Work out the finished part from the listing and answer in its coordinate system (mm). Coordinates: 2 decimals unless noted, no trailing zeros. Order: outer loops, then holes, each group sorted by start corner. A loop starts at its lowest first (then second) coordinate and runs counter-clockwise, first axis right, second up. Notation, with made-up numbers: (-4, 70) -> (22, 70) arc R19 cw to (22, 106) -> close; hole circle Ø9 at (81, -30.5). An arc over 180 degrees is marked (long way). Answer as CSV lines item,"result". Start each with the question number.
Item 1: Section D-D (z = -280.5) is taken. Write down the section's boundary in (x, y), then the cut area to 3 significant figures.
Item 2: Each of these flat-tipped pins is pushed along its axis until it touches: pin 1 Ø2 at (x, z) = (333.5, 118.5) entering from -Y; pin 2 Ø0.5 at (x, y) = (-524.5, 37) entering from +Z; pin 3 Ø8 at (y, z) = (11.5, 20) entering from +X. Where does it stop, or does it pass through?
Item 3: Straight lines are drawn through the part: L1, parallel to Z at x = 0, y = 65; L2, parallel to Y at x = 367, z = 51; L3, parallel to X at y = 33.5, z = 119. For each, find the intervals that lie inside material, in ascending order.
Item 4: Section B-B (z = 28) is taken. Write down the section's boundary in (x, y).
Item 5: Section C-C (y = 22) is taken. Write down the section's boundary in (x, z) (1 decimal), then the cut area to 3 significant figures.
Item 6: Section A-A (x = 0) is taken. Write down the section's boundary in (y, z), then the cut area to 3 significant figures.
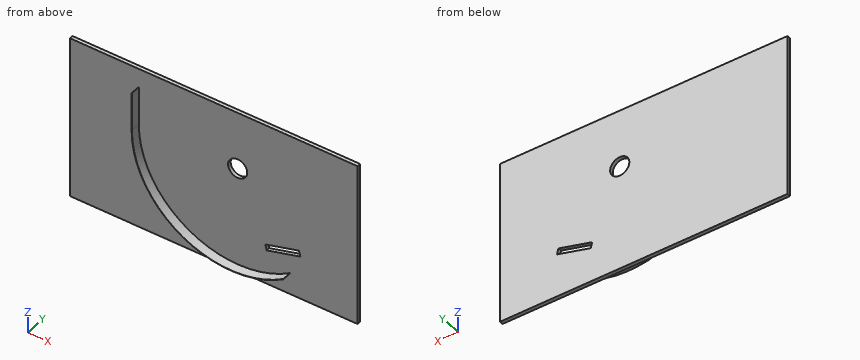
```python
from build123d import *

# Parameters (mm, degrees)
BOSS_EXTRUDE1_DEPTH    = 50.8
SKETCH4_W              = 1524
SKETCH4_H              = 863.6
BOSS_EXTRUDE2_DEPTH    = 19.05
F_20_0MM_DOWEL_HOLE1_D = 101.6
SKETCH8_W              = 1.5875
SKETCH8_H              = 50.8
BOSS_EXTRUDE3_DEPTH    = 204
CUT_EXTRUDE1_DEPTH     = 1052.265465998


with BuildPart() as part:
    # Sketch3 → Boss-Extrude1 (new body)
    with BuildSketch(Plane(origin=(0, 0, 0), x_dir=(1, 0, 0), z_dir=(0, 1, 0))):
        with BuildLine():
            Line((-524, 0), (-525.5875, 0))
            ThreePointArc((-525.5875, 0), (-255.243310314, 459.448661655), (277.677694458, 446.248045549))
            Line((277.677694458, 446.248045549), (277.677694458, 444.377202386))
            ThreePointArc((277.677694458, 444.377202386), (-254.040241009, 458.300726541), (-524, 0))
        make_face()
    extrude(amount=BOSS_EXTRUDE1_DEPTH)

    # Sketch4 → Boss-Extrude2 (add)
    with BuildSketch(Plane(origin=(0, 50.8, 0), x_dir=(1, 0, 0), z_dir=(0, 1, 0))):
        with Locations((-127, 127)):
            Rectangle(SKETCH4_W, SKETCH4_H)
    extrude(amount=BOSS_EXTRUDE2_DEPTH)

    # Ø20.0mm Dowel Hole1 (through all)
    with Locations(Plane(origin=(0, 50.8, 0), x_dir=(-1, 0, 0), z_dir=(0, -1, 0))):
        with Locations((0, 0)):
            Hole(F_20_0MM_DOWEL_HOLE1_D / 2)

    # Sketch8 → Boss-Extrude3 (add)
    with BuildSketch(Plane.XY):
        with Locations((-524.79375, 25.4)):
            Rectangle(SKETCH8_W, SKETCH8_H)
    extrude(amount=BOSS_EXTRUDE3_DEPTH)

    # Sketch9 → Cut-Extrude1 (cut, through all)
    with BuildSketch(Plane(origin=(0, 50.8, 0), x_dir=(-1, 0, 0), z_dir=(0, -1, 0))):
        Polygon((-154.06829349, 376.859298133), (-332.764571353, 328.977774789), (-325, 300), (-146.303722137, 347.881523344), align=None)
    extrude(amount=-CUT_EXTRUDE1_DEPTH, mode=Mode.SUBTRACT)


solid = part.part
```
Checked values:
1,outline,"(-889, 50.8) -> (-444.48, 50.8) -> (-444.48, 0) -> (-442.6, 0) -> (-442.6, 50.8) -> (635, 50.8) -> (635, 69.85) -> (-889, 69.85) -> close"
1,area,"29,100 mm^2"
2,pin 1,"stops at y = 50.8"
2,pin 2,"stops at z = 204"
2,pin 3,"stops at x = -524"
3,L1,"z = -558.8 to -50.8, 50.8 to 304.8"
3,L2,"y = 50.8 to 69.85"
3,L3,"x = -525.59 to -524"
4,outline,"(-889, 50.8) -> (-525.59, 50.8) -> (-525.59, 0) -> (-524, 0) -> (-524, 50.8) -> (-42.39, 50.8) -> (-42.39, 69.85) -> (-889, 69.85) -> close; (42.39, 50.8) -> (635, 50.8) -> (635, 69.85) -> (42.39, 69.85) -> close"
5,outline,"(-525.6, 0) arc R525.6 ccw to (277.7, -446.2) -> (277.7, -444.4) arc R524 cw to (-524, 0) -> (-524, 204) -> (-525.6, 204) -> close"
5,area,"2,100 mm^2"
6,outline,"(0, -525.59) -> (50.8, -525.59) -> (50.8, -558.8) -> (69.85, -558.8) -> (69.85, -50.8) -> (50.8, -50.8) -> (50.8, -524) -> (0, -524) -> close; (50.8, 50.8) -> (69.85, 50.8) -> (69.85, 304.8) -> (50.8, 304.8) -> close"
6,area,"14,600 mm^2"
